CAD build for the part. Positions are in the model's coordinates, mm. A direction names the side the tool comes from. Coordinates: 2 decimals unless noted, no trailing zeros. Loops run counter-clockwise (first coordinate to the right, second up) from the corner with the lowest first, then second, coordinate; pieces in that order, holes last. Notation, with made-up numbers: (-25.5, 41.5) -> (26.5, 41.5) arc R29 cw to (26.5, 76.5) -> close; hole circle Ø10 at (-10.5, 79.5). An arc over 180 degrees is marked (long way). Answer as a JSON object with one key per item and string values. Group by question number.
from build123d import *

# Parameters (mm, degrees)
SKETCH1_W           = 546.1
SKETCH1_H           = 279.4
BOSS_EXTRUDE1_DEPTH = 6.35
SKETCH2_W           = 31.75
SKETCH2_H           = 155.575
SKETCH2_W_2         = 6.35
SKETCH2_H_2         = 222.25
SKETCH2_W_3         = 63.5
SKETCH2_H_3         = 53.975
SKETCH2_W_4         = 495.3
SKETCH2_H_4         = 6.35
CUT_EXTRUDE1_DEPTH  = 307.975051918
EXTRUDE2_DEPTH      = 63.5
SKETCH4_R           = 25.4
BOSS_EXTRUDE2_DEPTH = 63.5


with BuildPart() as part:
    # Sketch1 → Boss-Extrude1 (new, symmetric)
    with BuildSketch(Plane(origin=(0, 0, 0), x_dir=(1, 0, 0), z_dir=(0, 1, 0))):
        Rectangle(SKETCH1_W, SKETCH1_H)
    extrude(amount=BOSS_EXTRUDE1_DEPTH, both=True)

    # Sketch2 → Cut-Extrude1 (cut, through all)
    with BuildSketch(Plane(origin=(0, 6.35, 0), x_dir=(1, 0, 0), z_dir=(0, 1, 0))):
        with Locations((0, -61.9125)):
            Rectangle(SKETCH2_W, SKETCH2_H)
        with Locations((-269.875, -28.575)):
            Rectangle(SKETCH2_W_2, SKETCH2_H_2)
        with Locations((53.975, -63.5)):
            Rectangle(SKETCH2_W_3, SKETCH2_H_3)
        with Locations((0, 136.525)):
            Rectangle(SKETCH2_W_4, SKETCH2_H_4)
        with Locations((269.875, -28.575)):
            Rectangle(SKETCH2_W_2, SKETCH2_H_2)
    extrude(amount=-CUT_EXTRUDE1_DEPTH, mode=Mode.SUBTRACT)

    # Sketch3 → Extrude2 (add)
    with BuildSketch(Plane.XZ.offset(6.35)):
        Polygon((222.25, -116.992783244), (129.182460015, -44.45), (-129.182460015, -44.45), (-222.25, -116.992783244), (-275.22182791, -136.272951858), (-273.05, -142.24), (-219.136547039, -122.617107896), (-127, -50.8), (127, -50.8), (219.136547039, -122.617107896), (273.05, -142.24), (275.22182791, -136.272951858), align=None)
    extrude(amount=EXTRUDE2_DEPTH)

    # Sketch4 → Boss-Extrude2 (add)
    with BuildSketch(Plane(origin=(0, 6.35, 0), x_dir=(1, 0, 0), z_dir=(0, 1, 0))):
        with Locations(Location((234.95, -107.95, 0), (0, 0, 90))):
            Circle(SKETCH4_R)
        with Locations(Location((-234.95, -107.95, 0), (0, 0, 90))):
            Circle(SKETCH4_R)
    extrude(amount=BOSS_EXTRUDE2_DEPTH)


solid = part.part
Item 1: Pull direction Z, two halves, no side cores. Call faces 1 (the flat face through (54, 0, 90.488)), 2 (the flat face through (-273.05, 0, -111)), 3 (the flat face through (0, 0, -15.875)): +Z half, -Z half, draft (parallel to the pull), parting line (faces both ways), or undercut.
Item 2: Band-saw the part on D-D, the plane y = -31.5. List the corners of the cut face in (x, z), and give its area (3 significant figures).
Item 3: Flat gauge pins, fed straight in: P1, Ø6.5, axis at y = 0.5, z = 31.5, coming from the -X side; P2, Ø5, axis at y = 2.5, z = -135.5, coming from the -X side; P3, Ø1, axis at x = -32.5, z = 82, coming from the -Y side. Where does each tip first touch, or does it go through?
Item 4: Drill centre lines: L1, parallel to Z at x = -92.5, y = -60.5; L2, parallel to Y at x = -114, z = -62; L3, parallel to X at y = -7, z = -74.5. Where is each one in solid material? Low to high.
Item 5: Band-saw the part on B-B, the plane x = 43. List the corners of the cut face in (y, z).
Item 6: 3-axis set-ups, long thin cutter, end or side, ignore diameter. For faces 4 (the flat face through (-248.37, -37.66, -126.5)), 5 (the flat face through (-266.7, 0, 30)), 6 (the flat face through (266.7, 0, 30)): which of +Z, -Z, +X, -X, +Y, -Y reach the whole face in a straight line?
Item 7: Band-saw the part on A-A, the plane z = 107.95. List the corners of the cut face in (x, y) (3 decimals).
Item 8: Band-saw the part on C-C, the plane z = 67. List the corners of the cut face in (x, y) (3 decimals).
Reply:
{
 "1": {"face 1": "undercut", "face 2": "draft", "face 3": "+Z half"},
 "2": {"outline": "(-275.22, -136.27) -> (-273.05, -142.24) -> (-219.14, -122.62) -> (-127, -50.8) -> (127, -50.8) -> (219.14, -122.62) -> (273.05, -142.24) -> (275.22, -136.27) -> (222.25, -116.99) -> (129.18, -44.45) -> (-129.18, -44.45) -> (-222.25, -116.99) -> close", "area": "3,840 mm²"},
 "3": {"P1": "x = -266.7", "P2": "x = -273.05", "P3": "y = -6.35"},
 "4": {"L1": "-50.8 to -44.45", "L2": "-6.35 to 6.35", "L3": "-167.73 to -157.41, 157.41 to 167.73"},
 "5": {"outline": "(-69.85, -50.8) -> (-6.35, -50.8) -> (-6.35, -133.35) -> (6.35, -133.35) -> (6.35, 36.51) -> (-6.35, 36.51) -> (-6.35, -44.45) -> (-69.85, -44.45) -> close; (-6.35, 90.49) -> (6.35, 90.49) -> (6.35, 139.7) -> (-6.35, 139.7) -> close"},
 "6": {"face 4": "+Z, -X, -Y", "face 5": "+Z, -X, +Y, -Y", "face 6": "+Z, +X, +Y, -Y"},
 "7": {"outline": "(-266.7, -6.35) -> (-15.875, -6.35) -> (-15.875, 6.35) -> (-209.55, 6.35) -> (-209.55, 69.85) -> (-260.35, 69.85) -> (-260.35, 6.35) -> (-266.7, 6.35) -> close; (15.875, -6.35) -> (266.7, -6.35) -> (266.7, 6.35) -> (260.35, 6.35) -> (260.35, 69.85) -> (209.55, 69.85) -> (209.55, 6.35) -> (15.875, 6.35) -> close"},
 "8": {"outline": "(-266.7, -6.35) -> (-15.875, -6.35) -> (-15.875, 6.35) -> (-266.7, 6.35) -> close; (15.875, -6.35) -> (22.225, -6.35) -> (22.225, 6.35) -> (15.875, 6.35) -> close; (85.725, -6.35) -> (266.7, -6.35) -> (266.7, 6.35) -> (85.725, 6.35) -> close"}
}
